Verification items for the finished model (mm, model axes). Face numbers are marked on the shaded views. Round coordinates to 2 decimals unless told otherwise and drop trailing zeros. Write each loop counter-clockwise with the first axis right and the second up, starting at its lowest first coordinate (ties: lowest second). Pieces come first, ordered by that corner, then holes.
from build123d import *

# Parameters (mm, degrees)
SKETCH_1_W          = 16
SKETCH_1_H          = 35
EXTRUDE_1_DEPTH     = 7
SKETCH_2_R          = 5.35
CUT_EXTRUDE_1_DEPTH = 1.3
SKETCH_3_R          = 4.5
CUT_EXTRUDE_2_DEPTH = 21.068383094
SKETCH_4_R          = 3
CUT_EXTRUDE_3_DEPTH = 2
SKETCH_6_R          = 2.25
CUT_EXTRUDE_4_DEPTH = 20.880895352


with BuildPart() as part:
    # 草图1 → 凸台-拉伸1 (new body)
    with BuildSketch(Plane(origin=(0, 0, 0), x_dir=(1, 0, 0), z_dir=(0, 1, 0))):
        Rectangle(SKETCH_1_W, SKETCH_1_H)
    extrude(amount=EXTRUDE_1_DEPTH)

    # 草图2 → 切除-拉伸1 (cut)
    with BuildSketch(Plane.XZ):
        with Locations(Location((0, 0, 0), (0, 0, 270))):
            Circle(SKETCH_2_R)
    extrude(amount=-CUT_EXTRUDE_1_DEPTH, mode=Mode.SUBTRACT)

    # 草图3 → 切除-拉伸2 (cut, through all)
    with BuildSketch(Plane.XZ.offset(-1.3)):
        with Locations(Location((0, 0, 0), (0, 0, 270))):
            Circle(SKETCH_3_R)
    extrude(amount=-CUT_EXTRUDE_2_DEPTH, mode=Mode.SUBTRACT)

    # 草图4 → 切除-拉伸3 (cut)
    with BuildSketch(Plane(origin=(0, 7, 0), x_dir=(1, 0, 0), z_dir=(0, 1, 0))):
        with Locations(Location((0, 11.5, 0), (0, 0, 270))):
            Circle(SKETCH_4_R)
        with Locations(Location((0, -11.5, 0), (0, 0, 270))):
            Circle(SKETCH_4_R)
    extrude(amount=-CUT_EXTRUDE_3_DEPTH, mode=Mode.SUBTRACT)

    # 草图6 → 切除-拉伸4 (cut, through all)
    with BuildSketch(Plane(origin=(0, 5, 0), x_dir=(1, 0, 0), z_dir=(0, 1, 0))):
        with Locations(Location((0, -11.5, 0), (0, 0, 270))):
            Circle(SKETCH_6_R)
        with Locations(Location((0, 11.5, 0), (0, 0, 270))):
            Circle(SKETCH_6_R)
    extrude(amount=-CUT_EXTRUDE_4_DEPTH, mode=Mode.SUBTRACT)


solid = part.part
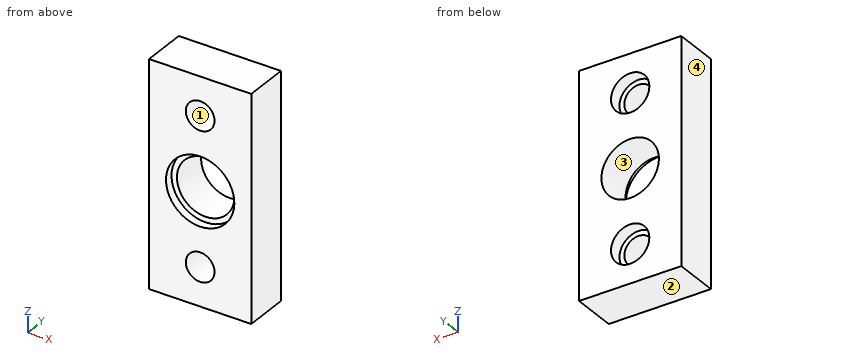
Q1. Sectioned sample at A-A (z = 0). Enter the section's corners in (x, y), plus the area to 3 significant figures.
Recorded:
outline: (-8, 0) - (-5.35, 0) - (-5.35, 1.3) - (-4.5, 1.3) - (-4.5, 7) - (-8, 7) - close; (4.5, 1.3) - (5.35, 1.3) - (5.35, 0) - (8, 0) - (8, 7) - (4.5, 7) - close
area: 46.8 mm2
Q2. Sectioned sample at C-C (x = 0). Enter the section's corners in (y, z).
Recorded:
outline: (0, -17.5) - (7, -17.5) - (7, -14.5) - (5, -14.5) - (5, -13.75) - (0, -13.75) - close; (0, -9.25) - (5, -9.25) - (5, -8.5) - (7, -8.5) - (7, -4.5) - (1.3, -4.5) - (1.3, -5.35) - (0, -5.35) - close; (0, 5.35) - (1.3, 5.35) - (1.3, 4.5) - (7, 4.5) - (7, 8.5) - (5, 8.5) - (5, 9.25) - (0, 9.25) - close; (0, 13.75) - (5, 13.75) - (5, 14.5) - (7, 14.5) - (7, 17.5) - (0, 17.5) - close
Q3. Sectioned sample at B-B (y = 5.5). Enter the section's corners in (x, z), plus the area to 3 significant figures.
Recorded:
outline: (-8, -17.5) - (8, -17.5) - (8, 17.5) - (-8, 17.5) - close; hole circle Ø9 at (0, 0); hole circle Ø6 at (0, -11.5); hole circle Ø6 at (0, 11.5)
area: 440 mm2
Q4. Release check for a two-part mould opening along Z. For the marked faces 1, 2, 3 and 4 record: released by +Z, released by -Z, zero draft, split by the parting line, or undercut.
Recorded:
face 1: undercut
face 2: released by -Z
face 3: undercut
face 4: zero draft
Q5. Sectioned sample at D-D (z = 11.5). Enter the section's corners in (x, y).
Recorded:
outline: (-8, 0) - (-2.25, 0) - (-2.25, 5) - (-3, 5) - (-3, 7) - (-8, 7) - close; (2.25, 0) - (8, 0) - (8, 7) - (3, 7) - (3, 5) - (2.25, 5) - close
Q6. Depth check by flat-ended pin: P1, Ø5.5, axis at x = 0, z = 0, coming from the -Y side. Enter the tip coordinate at first touch or a pass-through.
Recorded:
P1: passes through
Q7. Material ranges on line 1 along X through (y, z) = (5.65, -11.5); line 2 along X through (y, z) = (3.6, 11.5); line 3 along Z through (x, y) = (0.5, 4.5), recorded low to high.
Recorded:
line 1: x = -8 to -3, 3 to 8
line 2: x = -8 to -2.25, 2.25 to 8
line 3: z = -17.5 to -13.69, -9.31 to -4.47, 4.47 to 9.31, 13.69 to 17.5
